Build history of the part. All positions in model axes, mm. Face numbers are marked on the shaded views. A direction names the side the tool comes from. Coordinates: 2 decimals unless noted, no trailing zeros. Write each loop counter-clockwise with the first axis right and the second up, starting at its lowest first coordinate (ties: lowest second). Pieces come first, ordered by that corner, then holes. Notation, with made-up numbers: (-30.5, 9.25) -> (-8.5, 9.25) arc R16 ccw to (-8.5, 36.25) -> close; hole circle Ø5 at (-19, 13.5). An arc over 180 degrees is marked (long way). Write each question's results on one line, items separated by ' | '. Start each with the question number.
Q1. Saw through at A-A on x = 2.25. Give the cut face in (y, z), and give its area (3 significant figures).
Q2. Drill centre lines: line 1 (X direction, y = 0.1, z = -2.25); line 2 (Z direction, x = 10, y = 0); line 3 (Y direction, x = -0.75, z = 0.1). Where is each one in solid material? Low to high.
Q3. Two-plate mould, pull along Z, no slides. Class the marked faces 3, 4 and 5: released by +Z, released by -Z, zero draft, split by the parting line, or undercut.
Q4. Tool access for the marked faces 1 and 2: list every direction of +Z, -Z, +X, -X, +Y, -Y with a clear straight run to the whole face (end or side of a thin tool).
Q5. Drop flat-ended pins along their axis: pin 1 Ø2 at (x, y) = (3, 0) entering from -Z; pin 2 Ø3 at (x, y) = (5.5, 1.5) entering from +Z. Give the stop position or say it passes through.
Autodesk Inventor part; units mm, degrees
ref_plane "Work Plane1" through (29, 0, 0) normal (0, -1, 0) x (1, 0, 0)
ref_plane "YZ Plane" through (0, 0, 0) normal (1, 0, 0) x (0, 1, 0)
ref_plane "XZ Plane" through (0, 0, 0) normal (0, 1, 0) x (-1, 0, 0)
sketch "Sketch1" plane through (0, 0, 0) normal (0, 0, 1) x (1, 0, 0)
  line L0 (-0.8667, 0) -> (20, 0)
  line L1 (20, 0) -> (20, 1.5)
  line L2 (20, 1.5) -> (1.25, 1.5)
  line L3 (1.25, 1.5) -> (0.9432, 1.5)
  line L4 (0.9432, 1.5) -> (0, 1.5)
  line L5 (0, 1.5) -> (0, 2.75)
  line L6 (0, 2.75) -> (-3, 2.75)
  line L7 (-3, 2.75) -> (-3, 1.4434)
  line L8 (-3, 1.4434) -> (-1.7, 1.4434)
  line L9 (-1.7, 1.4434) -> (-0.8667, 0)
  line L10 (-7.6, 0) -> (24.6, 0)
  line L11 (0, -0.55) -> (0, 3.3)
  line L12 (1.25, 1.5) -> (0, 1.5) construction
  dimension "d1" = 18.75
  dimension "d2" = 0.3068
  dimension "d3" = 3
  dimension "d4" = 1.3
  dimension "d5" = 60
  dimension "d6" = 3
  dimension "d7" = 3
  dimension "d8" = 2.8868
  dimension "d9" = 5.5
  dimension "d26" = 20
revolve "Body" add sketch "Sketch1" angle 360 about axis through (-0.8667, 0, 0) along (1, 0, 0)
sketch "Sketch2" plane through (-3, 0, 0) normal (-1, 0, 0) x (0, 0, 1)
  circle A0 centre (0, 0) radius 1.4434
  line L0 (0, -3.85) -> (0, 3.85)
  line L1 (-3.85, 0) -> (3.85, 0)
  line L2 (1.4434, 0) -> (0.7217, -1.25)
  line L3 (0.7217, -1.25) -> (-0.7217, -1.25)
  line L4 (-0.7217, -1.25) -> (-1.4434, 0)
  line L5 (-1.4434, 0) -> (-0.7217, 1.25)
  line L6 (-0.7217, 1.25) -> (0.7217, 1.25)
  line L7 (0.7217, 1.25) -> (1.4434, 0)
  point P0 (0, 0)
extrude "Slot" add sketch "Sketch2" against normal up to next contours L7 A0 | A0 L2 | L6 L0 A0 | A0 L0 L3 | L0 L6 A0 | A0 L3 L0 | L4 A0 | A0 L5
fillet "Fillet1" radius 0.3 1 edges at (-3, -2.75, 0)
thread "Thread"
chamfer "Chamfer1" distance 0.3067 distance2 0.3067 1 edges at (20, -1.5, 0) measured on face at (20, -0.7567, -0.3972)
ref_plane "Work Plane1" through (29, 0, 0) normal (0, -1, 0) x (1, 0, 0)
fillet "Fillet2" radius 0.1 1 edges at (0, -1.5, 0)
equation "\"d1\" = GEL"
equation "\"d3\" = KOH"
equation "\"d4\" = INTI"
equation "\"d6\" = GD"
equation "\"d7\" = BDM"
equation "\"d8\" = 1.1547 * SW"
equation "\"d9\" = KOD"
equation "\"d26\" = NLG"
equation "\"d30\" = R"
equation "\"d17\" = RR"
equation "\"d13\" = GEL"
equation "\"d15\" = -0.5 * SPD + 0.5 * GD"
equation "\"d16\" = GUL"
equation "\"GD\" = NND"
equation "\"NLG\" = 20"
equation "\"GEL\" = 18.75"
equation "\"KOD\" = 5.5"
equation "\"KOH\" = 3"
equation "\"INTI\" = 1.3"
equation "\"GAL\" = 0.61345 * PTC"
equation "\"GUL\" = 0.61345 * PTC"
equation "\"BDM\" = NND"
equation "\"SW\" = 2.5"
equation "\"RR\" = 0.3"
equation "\"SPD\" = NND - 1.2269 * PTC"
equation "\"R\" = 0.1"
equation "\"TOA\" = 30deg"
equation "\"GD1\" = THREADDIA - 1.2269 * PTC"
equation "\"THREADDIA\" = 3"
equation "\"FAWI\" = 45deg"
equation "\"ANG\" = 120deg"
equation "\"PTC\" = 0.5"
equation "\"NND\" = 3"
equation "\"E0\" = 1.155 * SW"
properties part number "DIN 912 - M3 x 20" material "Steel, Mild"
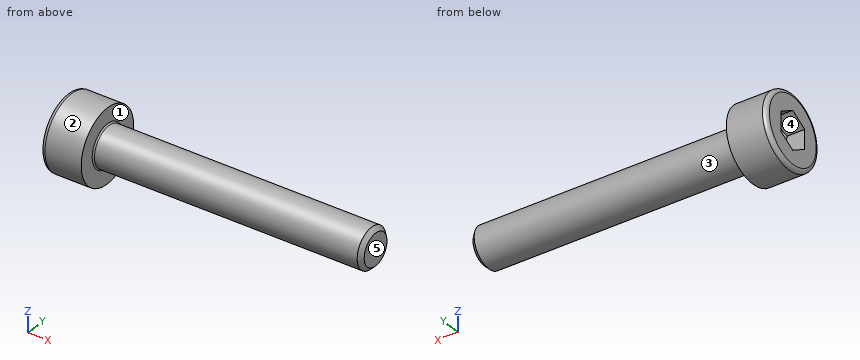
Returned:
1) outline: circle Ø3 at (0, 0) | area: 7.07 mm2
2) line 1: x = -3 to 0 | line 2: z = -1.5 to 1.5 | line 3: y = -2.75 to 2.75
3) face 3: split by the parting line | face 4: undercut | face 5: zero draft
4) face 1: +X | face 2: +X, -X
5) pin 1: stops at z = -1.5 | pin 2: stops at z = 1.5
